Read the model definition and answer for the solid it produces. Units are mm, in the model's axes. A direction names the side the tool comes from. Coordinates: 2 decimals unless noted, no trailing zeros. Write each loop counter-clockwise with the first axis right and the second up, starting at its lowest first coordinate (ties: lowest second). Pieces come first, ordered by that corner, then holes. Notation, with made-up numbers: (64.25, -23) - (74.25, -23) arc R20 ccw to (74.25, 13) - close; hole circle Ø11 at (78, 23). An arc over 180 degrees is marked (long way). Return JSON: item names as keys, results as strings.
```python
from build123d import *

# Parameters (mm, degrees)
SKETCH1_W           = 304.8
SKETCH1_H           = 152.4
BOSS_EXTRUDE1_DEPTH = 50.8
SHELL1_T            = -3.175
SKETCH3_W           = 12.7
SKETCH3_H           = 6.35
BOSS_EXTRUDE2_DEPTH = 6.35
SKETCH4_W           = 12.7
SKETCH4_H           = 6.35
BOSS_EXTRUDE3_DEPTH = 88.646
SKETCH5_W           = 12.7
SKETCH5_H           = 6.35
BOSS_EXTRUDE4_DEPTH = 3.81
CUT_EXTRUDE1_REACH  = 242.848


with BuildPart() as part:
    # Sketch1 → Boss-Extrude1 (new body)
    with BuildSketch(Plane.XY):
        with Locations((152.4, 76.2)):
            Rectangle(SKETCH1_W, SKETCH1_H)
    extrude(amount=BOSS_EXTRUDE1_DEPTH)

    # Shell1
    shell1_openings = [part.faces().sort_by_distance(p)[0] for p in [
        (152.4, 76.2, 0),
    ]]
    offset(amount=SHELL1_T, openings=shell1_openings, kind=Kind.INTERSECTION)

    # Sketch3 → Boss-Extrude2 (add)
    with BuildSketch(Plane(origin=(0, 152.4, 0), x_dir=(1, 0, 0), z_dir=(0, 1, 0))):
        with Locations((151.599627363, -3.175)):
            Rectangle(SKETCH3_W, SKETCH3_H)
    boss_extrude2 = extrude(amount=BOSS_EXTRUDE2_DEPTH)

    # Sketch4 → Boss-Extrude3 (add)
    with BuildSketch(Plane(origin=(0, 0, 0), x_dir=(-1, 0, 0), z_dir=(0, 0, -1))):
        with Locations((-151.599627363, 155.575)):
            Rectangle(SKETCH4_W, SKETCH4_H)
    boss_extrude3 = extrude(amount=BOSS_EXTRUDE3_DEPTH)

    # Sketch5 → Boss-Extrude4 (add)
    with BuildSketch(Plane.XZ.offset(-152.4)):
        with Locations((151.599627363, -85.471)):
            Rectangle(SKETCH5_W, SKETCH5_H)
    boss_extrude4 = extrude(amount=BOSS_EXTRUDE4_DEPTH)

    # Sketch6 → Cut-Extrude1 (cut, up to next)
    with BuildSketch(Plane(origin=(157.949627363, 0, 0), x_dir=(0, 0, -1), z_dir=(1, 0, 0)), mode=Mode.PRIVATE) as cut_extrude1_sk1:
        Polygon((83.385506006, 148.59), (88.646, 153.67), (88.646, 148.59), align=None)
    cut_extrude1_tool1 = extrude(cut_extrude1_sk1.sketch, amount=-CUT_EXTRUDE1_REACH, mode=Mode.PRIVATE) & part.part
    cut_extrude1 = cut_extrude1_tool1.solids().sort_by_distance((157.949627, 150.283333, -86.892502))[0]
    add(cut_extrude1, mode=Mode.SUBTRACT)

    # Mirror1: Boss-Extrude2, Boss-Extrude3, Boss-Extrude4, Cut-Extrude1 across plane
    add(boss_extrude2.mirror(Plane(origin=(0, 76.2, 0), x_dir=(0, 0, 1), z_dir=(0, -1, 0))))
    add(boss_extrude3.mirror(Plane(origin=(0, 76.2, 0), x_dir=(0, 0, 1), z_dir=(0, -1, 0))))
    add(boss_extrude4.mirror(Plane(origin=(0, 76.2, 0), x_dir=(0, 0, 1), z_dir=(0, -1, 0))))
    add(cut_extrude1.mirror(Plane(origin=(0, 76.2, 0), x_dir=(0, 0, 1), z_dir=(0, -1, 0))), mode=Mode.SUBTRACT)


solid = part.part
```
(1) A cutting plane is placed at A-A (z = -41.5). Determine the outline of the cut face in (x, y).
Answer:
{"outline": "(145.25, -6.35) - (157.95, -6.35) - (157.95, 0) - (145.25, 0) - close; (145.25, 152.4) - (157.95, 152.4) - (157.95, 158.75) - (145.25, 158.75) - close"}
(2) Determine the mould class of faces 5 (the face through (152, -6.35, -40)), 6 (the face through (145.25, 155, -42)), 7 (the face through (150, 3.175, 23)), 8 (the face through (3.175, 75, 23)) for opening direction X: +X half, -X half, draft (parallel to the pull), parting line (faces both ways), or undercut.
Answer:
{"face 5": "draft", "face 6": "-X half", "face 7": "undercut", "face 8": "undercut"}
(3) A cutting plane is placed at B-B (x = 197.5). Determine the outline of the cut face in (y, z) (3 decimals), and give its area (3 significant figures).
Answer:
{"outline": "(0, 0) - (3.175, 0) - (3.175, 47.625) - (149.225, 47.625) - (149.225, 0) - (152.4, 0) - (152.4, 50.8) - (0, 50.8) - close", "area": "786 mm²"}
(4) Straight lines are drawn through the part: line 1 (Y direction, x = 169.5, z = 34) (3 decimals); line 2 (X direction, y = 92, z = 16) (3 decimals); line 3 (Z direction, x = 157, y = 68) (3 decimals). For each, find the intervals that lie inside material, in ascending order. Write a range as from..to.
Answer:
{"line 1": "0..3.175, 149.225..152.4", "line 2": "0..3.175, 301.625..304.8", "line 3": "47.625..50.8"}
(5) A cutting plane is placed at C-C (z = 40.5). Determine the outline of the cut face in (x, y) (3 decimals).
Answer:
{"outline": "(0, 0) - (304.8, 0) - (304.8, 152.4) - (0, 152.4) - close; hole (3.175, 3.175) - (301.625, 3.175) - (301.625, 149.225) - (3.175, 149.225) - close"}
(6) Flat-ended cylindrical pins translate along their axes: P1, Ø24, axis at x = 223.5, z = 21.5, coming from the -Y side; P2, Ø14.5, axis at x = 206.5, z = 26.5, coming from the +Y side; P3, Ø11, axis at y = 153.5, z = -19.5, coming from the -X side; P4, Ø12, axis at x = 120.5, z = -8.5, coming from the +Y side. Find the tip coordinate at first contact, or state that the pin passes through.
Answer:
{"P1": "y = 0", "P2": "y = 152.4", "P3": "x = 145.25", "P4": "through"}
(7) Which of the six approach directions +Z, -Z, +X, -X, +Y, -Y give full straight-line access (tool end or side, diameter ignored) to faces 1 (the face through (152, 0, -41)), 2 (the face through (0, 75, 25)), 3 (the face through (152, -3, 6.35)), 4 (the face through (152, 156, 6.35))?
Answer:
{"face 1": "+X, -X", "face 2": "+Z, -Z, -X, +Y, -Y", "face 3": "+Z, +X, -X, -Y", "face 4": "+Z, +X, -X, +Y"}
(8) A cutting plane is placed at D-D (y = 8). Determine the outline of the cut face in (x, z) (3 decimals).
Answer:
{"outline": "(0, 0) - (3.175, 0) - (3.175, 47.625) - (301.625, 47.625) - (301.625, 0) - (304.8, 0) - (304.8, 50.8) - (0, 50.8) - close"}
